Model file for the job. Use its own axes, mm. A direction names the side the tool comes from. Round coordinates to 2 decimals unless told otherwise and drop trailing zeros. Order: outer loops, then holes, each group sorted by start corner. A loop starts at its lowest first (then second) coordinate and runs counter-clockwise, first axis right, second up. Notation, with made-up numbers: (44.25, -13) -> (85.25, -13) arc R14 cw to (85.25, 3) -> close; hole circle Ø3 at (21.25, 9.25). An arc over 180 degrees is marked (long way). Answer as CSV lines item,"result".
```python
from build123d import *

# Parameters (mm, degrees)
SKETCH1_W                = 4.5
SKETCH1_H                = 3.5
BOSS_EXTRUDE1_DEPTH      = 10
SKETCH2_W                = 3
SKETCH2_H                = 2
BOSS_EXTRUDE2_DEPTH      = 10.01
BOSS_EXTRUDE2_DEPTH_BACK = 0.01
FILLET2_R                = 0.5
SKETCH14_R               = 0.35


with BuildPart() as part:
    # Sketch1 → Boss-Extrude1 (new body)
    with BuildSketch(Plane(origin=(0, 0, 0), x_dir=(1, 0, 0), z_dir=(0, 1, 0))):
        Rectangle(SKETCH1_W, SKETCH1_H)
    extrude(amount=BOSS_EXTRUDE1_DEPTH)

    # Sketch2 → Boss-Extrude2 (add, two sides)
    with BuildSketch(Plane(origin=(0, 0, 0), x_dir=(1, 0, 0), z_dir=(0, 1, 0))) as boss_extrude2_sk:
        Rectangle(SKETCH2_W, SKETCH2_H)
    extrude(amount=BOSS_EXTRUDE2_DEPTH)
    extrude(boss_extrude2_sk.sketch, amount=-BOSS_EXTRUDE2_DEPTH_BACK)

    # Fillet2
    fillet2_edges = [part.edges().sort_by_distance(p)[0] for p in [
        (2.25, 5, 1.75),
        (-2.25, 5, 1.75),
        (-2.25, 5, -1.75),
        (2.25, 5, -1.75),
    ]]
    fillet(fillet2_edges, radius=FILLET2_R)

    # Sweep1: sweep along a path in Sketch15
    with BuildLine(Plane.XY) as sweep1_path:
        Line((2.25, 6.5), (2.3, 6.5))
        Line((2.3, 6.5), (2.525918375, 6.5))
        ThreePointArc((2.525918375, 6.5), (2.879471766, 6.353553391), (3.025918375, 6))
        Line((3.025918375, 6), (3.025918375, -71.146217922))
    # Sketch14 → Sweep1 (sweep)
    with BuildSketch(Plane(origin=(2.25, 0, 0), x_dir=(0, 0, -1), z_dir=(1, 0, 0))):
        with Locations((0, 6.5)):
            Circle(SKETCH14_R)
    sweep1 = sweep(path=sweep1_path.line)

    # Mirror1: Sweep1 across plane
    add(sweep1.mirror(Plane(origin=(0, 0, 0), x_dir=(0, 0, 1), z_dir=(1, 0, 0))))


solid = part.part
```
Q1. Tool access for faces 3 (the flat face through (0, -0.01, 0)), 4 (the flat face through (0, 5, -1.75)): list every direction of +Z, -Z, +X, -X, +Y, -Y with a clear straight run to the whole face (end or side of a thin tool).
Checks:
face 3,"+Z, -Z, -Y"
face 4,"-Z, +X, -X, +Y, -Y"
Q2. Wall check: L1, parallel to Y at x = 0.5, z = 0.6; L2, parallel to X at y = -49, z = 0.1; L3, parallel to X at y = -4.5, z = -0.3. Give the ranges that are in metal, low to high. Write a range as [from, to].
Checks:
L1,"[-0.01, 10.01]"
L2,"[-3.36, -2.69], [2.69, 3.36]"
L3,"[-3.21, -2.85], [2.85, 3.21]"
Q3. Saw through at B-B (y = -44). Write the cut outline in (x, z).
Checks:
outline,"circle Ø0.7 at (-3.03, 0); circle Ø0.7 at (3.03, 0)"
Q4. Mould opens along X. For faces 1 (the flat face through (0, 5, 1.75)), 2 (the flat face through (-2.25, 5, 0)) say: +X half, -X half, draft (parallel to the pull), parting line (faces both ways), or undercut.
Checks:
face 1,"draft"
face 2,"undercut"
Q5. Flat gauge pins, fed straight in: pin 1 (1.6 mm diameter, centred on x = -0.5, z = -0.5, fed in from -Y); pin 2 (1.5 mm diameter, centred on x = 2.5, z = 0, fed in from +Y); pin 3 (1 mm diameter, centred on x = -2, y = -46, fed in from +Z); pin 4 (4 mm diameter, centred on x = 1, y = -47.5, fed in from +Z). Where does each tip first touch, or does it go through?
Checks:
pin 1,"y = -0.01"
pin 2,"y = 10"
pin 3,"through"
pin 4,"z = 0.35"
